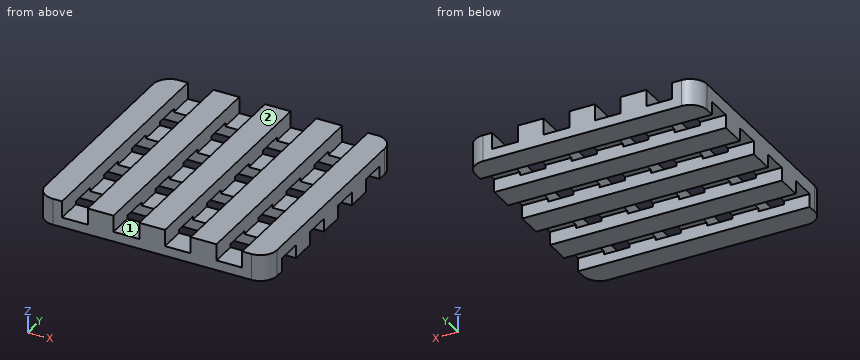
from build123d import *

# Parameters (mm, degrees)
F0_W     = 88.9
F0_H     = 10.16
F1_DEPTH = 88.9
F2_R     = 6.35
F3_W     = 9.877778
F3_H     = 6.35
F4_DEPTH = 88.901
F5_W     = 9.877778
F5_H     = 5.08
F6_DEPTH = 88.901


with BuildPart() as f1:
    # F0 (on Front) → F1 (new body)
    with BuildSketch(Plane.XZ):
        Rectangle(F0_W, F0_H)
    extrude(amount=F1_DEPTH)

    # F2
    f2_edges = [f1.edges().sort_by_distance(p)[0] for p in [
        (-44.45, -88.9, 0),
        (44.45, -88.9, 0),
        (44.45, 0, 0),
        (-44.45, 0, 0),
    ]]
    fillet(f2_edges, radius=F2_R)

    # F3 (on face) → F4 (cut, through all)
    with BuildSketch(Plane.XZ.offset(88.9)):
        with Locations((-29.633333, 1.905)):
            Rectangle(F3_W, F3_H)
        with Locations((-9.877778, 1.905)):
            Rectangle(F3_W, F3_H)
        with Locations((9.877778, 1.905)):
            Rectangle(F3_W, F3_H)
        with Locations((29.633333, 1.905)):
            Rectangle(F3_W, F3_H)
    extrude(amount=-F4_DEPTH, mode=Mode.SUBTRACT)

    # F5 (on face) → F6 (cut, through all)
    with BuildSketch(Plane.YZ.offset(44.45)):
        with Locations((-14.816667, -2.54)):
            Rectangle(F5_W, F5_H)
        with Locations((-34.572222, -2.54)):
            Rectangle(F5_W, F5_H)
        with Locations((-54.327778, -2.54)):
            Rectangle(F5_W, F5_H)
        with Locations((-74.083333, -2.54)):
            Rectangle(F5_W, F5_H)
    extrude(amount=-F6_DEPTH, mode=Mode.SUBTRACT)


solid = f1.part
Verification items for the finished model (mm, model axes). Face numbers are marked on the shaded views. A direction names the side the tool comes from. Coordinates: 2 decimals unless noted, no trailing zeros. Order: outer loops, then holes, each group sorted by start corner. A loop starts at its lowest first (then second) coordinate and runs counter-clockwise, first axis right, second up.
1. Go/stop test with flat-tipped pins: pin 1 Ø8 at (x, y) = (-0.5, -54.5) entering from -Z; pin 2 Ø3 at (x, y) = (9.5, -64.5) entering from +Z. Record where each tip stops, or that it passes through.
Results found:
pin 1: stops at z = 0
pin 2: stops at z = -1.27
2. Sectioned sample at A-A, the plane y = -51. Record the cut outline in (x, z), and give its area (3 significant figures).
Results found:
outline: (-44.45, 0) - (-34.57, 0) - (-34.57, 5.08) - (-44.45, 5.08) - close; (-24.69, 0) - (-14.82, 0) - (-14.82, 5.08) - (-24.69, 5.08) - close; (-4.94, 0) - (4.94, 0) - (4.94, 5.08) - (-4.94, 5.08) - close; (14.82, 0) - (24.69, 0) - (24.69, 5.08) - (14.82, 5.08) - close; (34.57, 0) - (44.45, 0) - (44.45, 5.08) - (34.57, 5.08) - close
area: 251 mm2
3. Scan lines: line 1 (Y direction, x = 21, z = -4.5); line 2 (X direction, y = -74.5, z = 3.75). Record each from-to range of solid material in increasing order.
Results found:
line 1: y = -88.9 to -79.02, -69.14 to -59.27, -49.39 to -39.51, -29.63 to -19.76, -9.88 to 0
line 2: x = -44.45 to -34.57, -24.69 to -14.82, -4.94 to 4.94, 14.82 to 24.69, 34.57 to 44.45
4. Set-up check for the marked faces 1 and 2: record each of +Z, -Z, +X, -X, +Y, -Y from which the full face is reachable in a straight line by a thin tool's end or side.
Results found:
face 1: +Z, +Y, -Y
face 2: +Z, +X, -X, +Y, -Y
5. Sectioned sample at D-D, the plane y = -65. Record the cut outline in (x, z).
Results found:
outline: (-44.45, -5.08) - (44.45, -5.08) - (44.45, 5.08) - (34.57, 5.08) - (34.57, -1.27) - (24.69, -1.27) - (24.69, 5.08) - (14.82, 5.08) - (14.82, -1.27) - (4.94, -1.27) - (4.94, 5.08) - (-4.94, 5.08) - (-4.94, -1.27) - (-14.82, -1.27) - (-14.82, 5.08) - (-24.69, 5.08) - (-24.69, -1.27) - (-34.57, -1.27) - (-34.57, 5.08) - (-44.45, 5.08) - close
6. Sectioned sample at B-B, the plane z = 3.5. Record the cut outline in (x, y), and give its area (3 significant figures).
Results found:
outline: (-44.45, -82.55) arc R6.35 ccw to (-38.1, -88.9) - (-34.57, -88.9) - (-34.57, 0) - (-38.1, 0) arc R6.35 ccw to (-44.45, -6.35) - close; (-24.69, -88.9) - (-14.82, -88.9) - (-14.82, 0) - (-24.69, 0) - close; (-4.94, -88.9) - (4.94, -88.9) - (4.94, 0) - (-4.94, 0) - close; (14.82, -88.9) - (24.69, -88.9) - (24.69, 0) - (14.82, 0) - close; (34.57, -88.9) - (38.1, -88.9) arc R6.35 ccw to (44.45, -82.55) - (44.45, -6.35) arc R6.35 ccw to (38.1, 0) - (34.57, 0) - close
area: 4,360 mm2
7. Sectioned sample at C-C, the plane x = 10.5. Record the cut outline in (y, z).
Results found:
outline: (-88.9, -5.08) - (-79.02, -5.08) - (-79.02, -1.27) - (-88.9, -1.27) - close; (-69.14, -5.08) - (-59.27, -5.08) - (-59.27, -1.27) - (-69.14, -1.27) - close; (-49.39, -5.08) - (-39.51, -5.08) - (-39.51, -1.27) - (-49.39, -1.27) - close; (-29.63, -5.08) - (-19.76, -5.08) - (-19.76, -1.27) - (-29.63, -1.27) - close; (-9.88, -5.08) - (0, -5.08) - (0, -1.27) - (-9.88, -1.27) - close
